Input: dimensioned drawing with shaded views. Units: mm. Origin: part minimum x, y, z. Coordinates: 2 decimals unless noted, no trailing zeros. Write each loop counter-clockwise with the first axis right and the second up, starting at its lowest first coordinate (ties: lowest second). Pieces come first, ordered by that corner, then holes. Notation, with made-up numbers: (-27, 66.5) -> (28, 66.5) arc R23 cw to (28, 74.5) -> close; hole circle Ø9 at (-3.5, -1). An arc over 180 degrees is marked (long way). One line per item, written item: value. Start each with the question number.
1. Mould query, pull axis Z, two halves, no side actions, for the marked faces 1, 2 and 3. Classes: released by +Z, released by -Z, zero draft, split by the parting line, or undercut.
2. First-contact query: P1, Ø2, axis at x = 53.5, z = 42, coming from the -Y side. Flat tip, straight axial feed; report the tip coordinate or a pass-through.
3. Section query C-C, the plane z = 43. Output: boundary loops of the cut face in (x, y), and give its area (3 significant figures).
4. Line query: line 1 (Z direction, x = 43, y = 4.8); line 2 (Z direction, x = 34.5, y = 0.6); line 3 (X direction, y = 1.7, z = 37.5). Output: solid intervals per line, ascending.
5. Section query B-B, the plane y = 4.75. Output: boundary loops of the cut face in (x, z), and give its area (3 significant figures).
6. Section query A-A, the plane x = 43. Output: boundary loops of the cut face in (y, z).
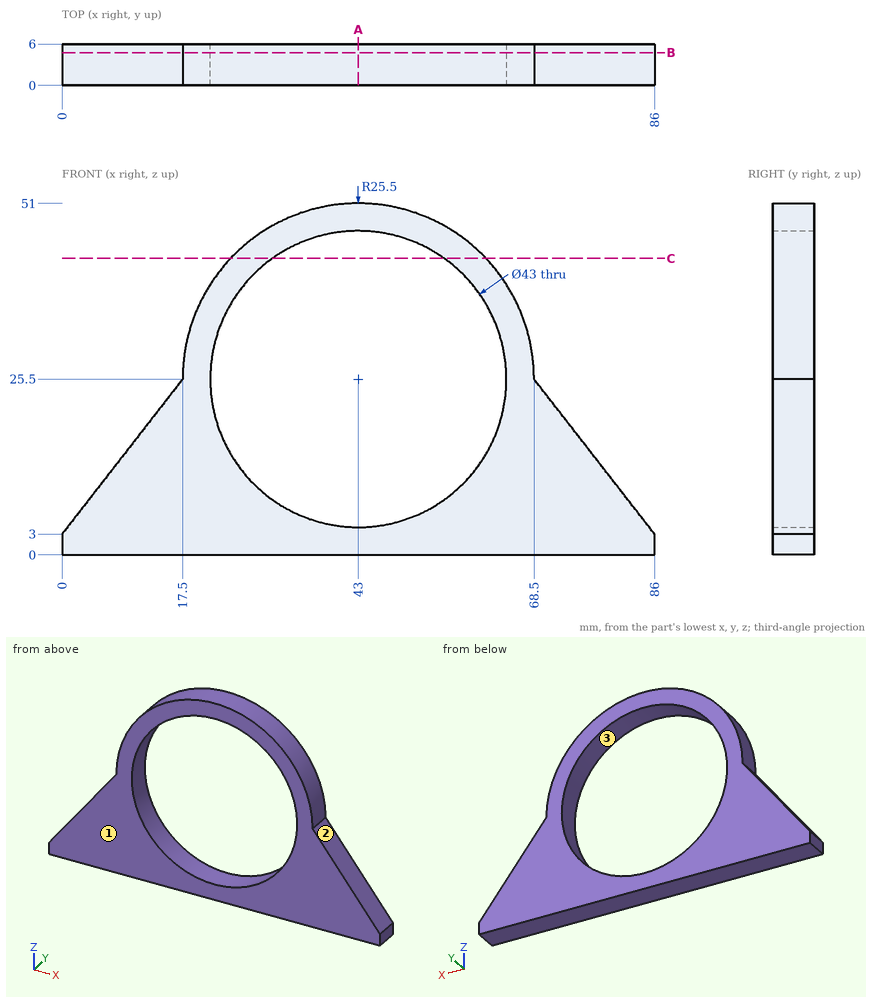
Computed values:
1. face 1: zero draft
1. face 2: released by +Z
1. face 3: undercut
2. P1: passes through
3. outline: (24.45, 0) -> (30.51, 0) -> (30.51, 6) -> (24.45, 6) -> close; (55.49, 0) -> (61.55, 0) -> (61.55, 6) -> (55.49, 6) -> close
3. area: 72.7 mm²
4. line 1: z = 0 to 4, 47 to 51
4. line 2: z = 0 to 5.75, 45.25 to 49.54
4. line 3: x = 20.5 to 25.16, 60.84 to 65.5
5. outline: (0, 0) -> (86, 0) -> (86, 3) -> (68.5, 25.5) arc R25.5 ccw to (17.5, 25.5) -> (0, 3) -> close; hole circle Ø43 at (43, 25.5)
5. area: 1,370 mm²
6. outline: (0, 0) -> (6, 0) -> (6, 4) -> (0, 4) -> close; (0, 47) -> (6, 47) -> (6, 51) -> (0, 51) -> close
